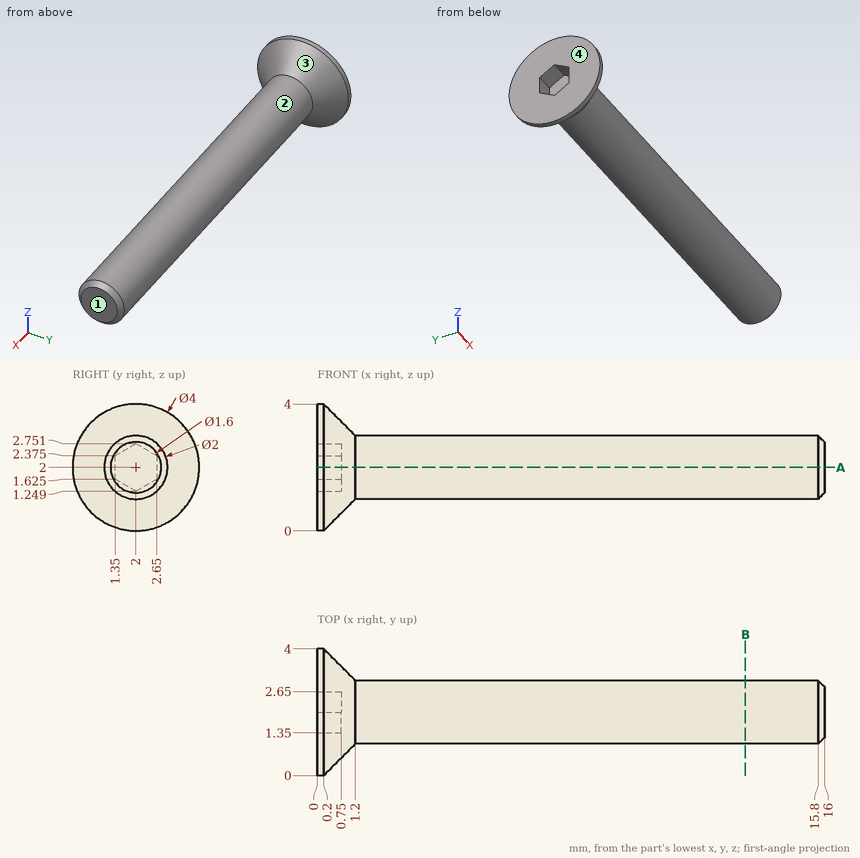
Geometry check sheet. Reference: drawing and pictorial views, mm from the part's lowest x, y, z. A direction names the side the tool comes from. Round coordinates to 2 decimals unless told otherwise and drop trailing zeros. Loops run counter-clockwise (first coordinate to the right, second up) from the corner with the lowest first, then second, coordinate; pieces in that order, holes last. Notation, with made-up numbers: (82.25, 42.5) - (123.25, 42.5) arc R24 cw to (123.25, 55.5) - close; hole circle Ø1 at (-30.75, 8.25). An arc over 180 degrees is marked (long way). Write item = value, one per line. Start each with the question number.
Q1. Access from +Z, -Z, +X, -X, +Y, -Y to the whole of each face (thin tool, end or side, straight path). Record for the marked faces 1 and 2.
Q2. Thickness scan on L1, parallel to X at y = 1.4, z = 2.3; L2, parallel to Z at x = 4, y = 1.4; L3, parallel to X at y = 1, z = 0.6. Record the ranges inside material, lowest first.
Q3. Depth check by flat-ended pin: P1, Ø2, axis at y = 0.5, z = 0.5, coming from the -X side. Enter the tip coordinate at first touch or a pass-through.
Q4. Section check A-A (z = 2). Record the boundary of the cut face in (x, y).
Q5. Release check for a two-part mould opening along Z. For the marked faces 3 and 4 record: pulls with the +Z half, pulls with the -Z half, needs draft (parallel to the pull), parting line crosses it, or undercut.
Q6. Section check B-B (x = 13.5). Record the boundary of the cut face in (y, z).
Derived:
q1.face_1 = +Z, -Z, +X, +Y, -Y
q1.face_2 = +X
q2.L1 = 0.75 to 16
q2.L2 = 1.2 to 2.8
q2.L3 = 0 to 0.48
q3.P1 = 0
q4.outline = (0, 0) - (0.2, 0) - (1.2, 1) - (15.8, 1) - (16, 1.2) - (16, 2.8) - (15.8, 3) - (1.2, 3) - (0.2, 4) - (0, 4) - (0, 2.65) - (0.75, 2.65) - (0.75, 1.35) - (0, 1.35) - close
q5.face_3 = parting line crosses it
q5.face_4 = needs draft
q6.outline = circle Ø2 at (2, 2)
